The figure shows three views and two pictorial views of one solid part (mm, origin at its lowest corner). Answer the questions. Coordinates: 2 decimals unless noted, no trailing zeros. Loops run counter-clockwise (first coordinate to the right, second up) from the corner with the lowest first, then second, coordinate; pieces in that order, holes last. Notation, with made-up numbers: M 45,56 L 62,56 A26 ccw 62,95 Z; hole C 1.25,-16 d3. An arc over 180 degrees is marked long. Answer in a Markdown table with one row per item. Add a question column.
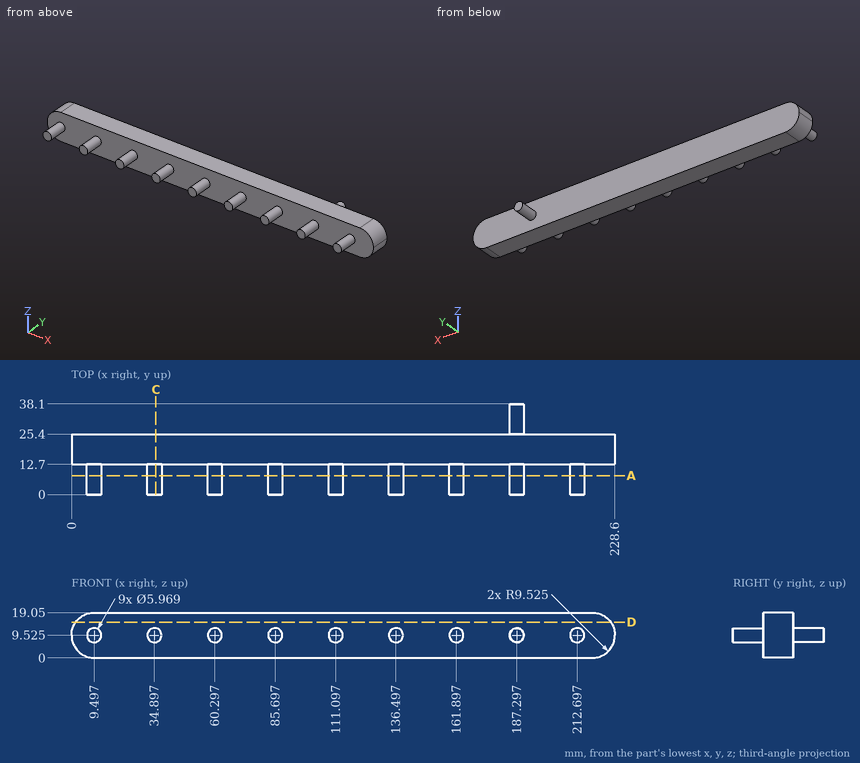
(1) Each of these flat-tipped pins is pushed along its axis until it touches: pin 1 (2 mm diameter, centred on y = 31.5, z = 15.5, fed in from -X); pin 2 (4 mm diameter, centred on x = 149, z = 3.5, fed in from -Y). Where does it stop, or does it pass through?
(2) A cutting plane is placed at D-D (z = 15). Give the vertices of the cut face in (x, y).
(3) A cutting plane is placed at A-A (y = 8). State how many separate pieces and enclosed holes the cut face has, plus the area to 3 significant figures.
(4) A cutting plane is placed at C-C (x = 35.5). Give the vertices of the cut face in (y, z).
(5) Straight lines are drawn through the part: line 1 (Y direction, x = 189, z = 4.5); line 2 (X direction, y = 28, z = 9.5); line 3 (X direction, y = 15, z = 9). For each, find the intervals that lie inside material, in ascending order.
Solved:
| question | item | result |
|---|---|---|
| 1 | pin 1 | passes through |
| 1 | pin 2 | stops at y = 12.7 |
| 2 | outline | M 1.73,12.7 L 226.87,12.7 L 226.87,25.4 L 1.73,25.4 Z |
| 3 | separate pieces | 9 |
| 3 | enclosed holes | 0 |
| 3 | area | 252 mm² |
| 4 | outline | M 0,6.6 L 12.7,6.6 L 12.7,0 L 25.4,0 L 25.4,19.05 L 12.7,19.05 L 12.7,12.45 L 0,12.45 Z |
| 5 | line 1 | y = 12.7 to 25.4 |
| 5 | line 2 | x = 184.31 to 190.28 |
| 5 | line 3 | x = 0.01 to 228.59 |
